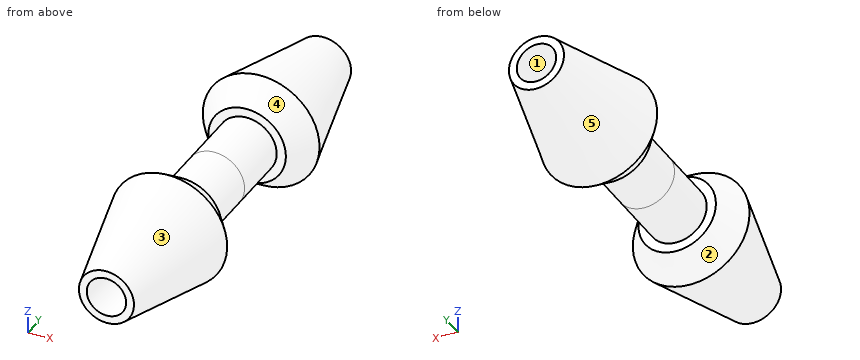
from build123d import *

# Parameters (mm, degrees)
CHAMFER1_SIZE       = 4.28
CHAMFER1_SIZE2      = 4.038825392
SKETCH8_R           = 4.5
BOSS_EXTRUDE2_DEPTH = 9.5
SKETCH9_R           = 3
CUT_EXTRUDE2_DEPTH  = 66.414452097


with BuildPart() as part:
    # Sketch7 → Revolve1 (revolve)
    with BuildSketch(Plane(origin=(0, 0, 0), x_dir=(0, 0, -1), z_dir=(1, 0, 0))):
        Polygon((0, 0), (0, 22.597995894), (4.193169033, 22.597995894), (9.941146123, 0), align=None)
    revolve(axis=Axis((0, 0, 0), (0, 1, 0)))

    # Chamfer1
    chamfer1_edges = [part.edges().sort_by_distance(p)[0] for p in [
        (0, 0, 9.941146123),
    ]]
    chamfer1_side = [part.faces().sort_by_distance(p)[0] for p in [
        (0, 11.298997947, 7.067157578),
    ]]
    chamfer(chamfer1_edges, length=CHAMFER1_SIZE, length2=CHAMFER1_SIZE2, reference=chamfer1_side[0])

    # Sketch8 → Boss-Extrude2 (add)
    with BuildSketch(Plane.XZ):
        with Locations(Location((0, 0, 0), (0, 0, 270))):
            Circle(SKETCH8_R)
    extrude(amount=BOSS_EXTRUDE2_DEPTH)

    # Mirror3: part across plane


with BuildPart() as part_1:
    add(part.part)
    add(part.part.mirror(Plane(origin=(0, -9.5, 0), x_dir=(0, 0, 1), z_dir=(0, -1, 0))))

    # Sketch9 → Cut-Extrude2 (cut, through all)
    with BuildSketch(Plane(origin=(0, 22.597995894, 0), x_dir=(1, 0, 0), z_dir=(0, 1, 0))):
        with Locations(Location((0, 0, 0), (0, 0, 270))):
            Circle(SKETCH9_R)
    extrude(amount=-CUT_EXTRUDE2_DEPTH, mode=Mode.SUBTRACT)


solid = part_1.part
Check sheet for the modelled part. Datum: model origin and axes. Units: mm. Face numbers are marked on the shaded views. A direction names the side the tool comes from. Round coordinates to 2 decimals unless told otherwise and drop trailing zeros. Write each loop counter-clockwise with the first axis right and the second up, starting at its lowest first coordinate (ties: lowest second). Pieces come first, ordered by that corner, then holes. Notation, with made-up numbers: (23.5, -22) - (63.5, -22) arc R18 cw to (63.5, -17) - close; hole circle Ø5 at (-39, 22.5). An arc over 180 degrees is marked (long way). Return JSON: item names as keys, results as strings.
Q1. Access from +Z, -Z, +X, -X, +Y, -Y to the whole of each face (thin tool, end or side, straight path). Record for the marked faces 1 and 2.
Returned:
{"face 1": "+Y, -Y", "face 2": "none"}
Q2. Depth check by flat-ended pin: P1, Ø6, axis at x = -6, y = -28.5, coming from the -Z side; P2, Ø10, axis at x = 6, y = -18, coming from the +Z side; P3, Ø10, axis at x = -3.5, y = -6, coming from the +Z side. Enter the tip coordinate at first touch or a pass-through.
Returned:
{"P1": "stops at z = -7.14", "P2": "stops at z = 7.52", "P3": "stops at z = 4.5"}
Q3. Cross-section at D-D (y = 6). Record the boundary of the cut face in (x, z) (3 decimals).
Returned:
{"outline": "circle Ø16.83 at (0, 0); hole circle Ø6 at (0, 0)"}
Q4. Draft check along Y on the marked faces 3, 4 and 5. Enter one of: released by +Y, released by -Y, zero draft, split by the parting line, or undercut.
Returned:
{"face 3": "released by -Y", "face 4": "undercut", "face 5": "released by +Y"}
Q5. Cross-section at C-C (y = -8.5). Record the boundary of the cut face in (x, z), then the cut area to 3 significant figures.
Returned:
{"outline": "circle Ø9 at (0, 0); hole circle Ø6 at (0, 0)", "area": "35.3 mm²"}
Q6. Cross-section at B-B (z = 0). Record the boundary of the cut face in (x, y), then the cut area to 3 significant figures.
Returned:
{"outline": "(-8.89, -23.15) - (-4.19, -41.6) - (-3, -41.6) - (-3, 22.6) - (-4.19, 22.6) - (-8.89, 4.15) - (-5.9, 0) - (-4.5, 0) - (-4.5, -19) - (-5.9, -19) - close; (3, -41.6) - (4.19, -41.6) - (8.89, -23.15) - (5.9, -19) - (4.5, -19) - (4.5, 0) - (5.9, 0) - (8.89, 4.15) - (4.19, 22.6) - (3, 22.6) - close", "area": "391 mm²"}
Q7. Cross-section at A-A (x = 0). Record the boundary of the cut face in (y, z).
Returned:
{"outline": "(-41.6, -4.19) - (-23.15, -8.89) - (-19, -5.9) - (-19, -4.5) - (0, -4.5) - (0, -5.9) - (4.15, -8.89) - (22.6, -4.19) - (22.6, -3) - (-41.6, -3) - close; (-41.6, 3) - (22.6, 3) - (22.6, 4.19) - (4.15, 8.89) - (0, 5.9) - (0, 4.5) - (-19, 4.5) - (-19, 5.9) - (-23.15, 8.89) - (-41.6, 4.19) - close"}
Q8. Scan lines: L1, parallel to X at y = -6, z = 0; L2, parallel to X at y = -22, z = 0; L3, parallel to Z at x = -6.5, y = 8. Record each from-to range of solid material in increasing order. Write a range as from..to.
Returned:
{"L1": "x = -4.5..-3, 3..4.5", "L2": "x = -8.06..-3, 3..8.06", "L3": "z = -4.5..4.5"}
